```python
from build123d import *

# Parameters (mm, degrees)
F1_DEPTH = 12.7
F2_R     = 1.8288
F3_DEPTH = 5.08


# Not quite as in the source:
# - the program builds the solid bodies; features that only make, move or delete a surface that nothing else refers to are left out


with BuildPart() as f1:
    # F0 (on Top) → F1 (new body)
    with BuildSketch(Plane.XY):
        Polygon((48.4242066741, -22.2311150283), (0, 52.6062995195), (-47.3236590624, -22.2311150283), align=None)
    extrude(amount=F1_DEPTH)

    # F2 (on face) → F3 (cut)
    with BuildSketch(Plane.XY.offset(12.7)):
        with Locations((-41.0783812404, -18.9761463553)):
            Circle(F2_R)
        with Locations((-20.4600691795, -18.9761463553)):
            Circle(F2_R)
        with Locations((0, -18.9761463553)):
            Circle(F2_R)
        with Locations((19.8642425239, -18.9761463553)):
            Circle(F2_R)
        with Locations((38.6579222977, -18.9761463553)):
            Circle(F2_R)
        with Locations((-29.1365217417, 3.3634696156)):
            Circle(F2_R)
        with Locations((-11.6957994178, 3.3634696156)):
            Circle(F2_R)
        with Locations((4.2915293016, 3.3634696156)):
            Circle(F2_R)
        with Locations((22.6406212896, 3.3634696156)):
            Circle(F2_R)
        with Locations((-15.87430574, 24.0743272007)):
            Circle(F2_R)
        with Locations((0, 24.0743272007)):
            Circle(F2_R)
        with Locations((13.3752385154, 24.0743272007)):
            Circle(F2_R)
        with Locations((-5.3372029215, 40.4250063002)):
            Circle(F2_R)
        with Locations((4.2915293016, 40.4250063002)):
            Circle(F2_R)
        with Locations((0, 48.2369959354)):
            Circle(F2_R)
    extrude(amount=-F3_DEPTH, mode=Mode.SUBTRACT)


solid = f1.part
```
Can you work these out from the model? Positions are in its coordinate system, mm. A direction names the side the tool comes from. Coordinates: 2 decimals unless noted, no trailing zeros. Loops run counter-clockwise (first coordinate to the right, second up) from the corner with the lowest first, then second, coordinate; pieces in that order, holes last. Notation, with made-up numbers: M 34,77.25 L 38,77.25 A19 ccw 38,88.25 Z; hole C 85.5,-1 d10. An arc over 180 degrees is marked long. Put each result on its own line as item: value. Start each with the question number.
(1) We'd pull the mould along Y, two halves only. Please class faces 3 (the face through (20, -19, 7.62)), 4 (the face through (-0.24, 50.05, 10.2)), 5 (the face through (0, -22.231, 6)), 6 (the face through (-23.33, 15.71, 6.26)): +Y half, -Y half, draft (parallel to the pull), parting line (faces both ways), or undercut.
(2) Imagine slicing it at A-A on z = 9.5. Give the number of separate pieces and of enclosed holes in the cut face, and give its area (3 significant figures).
(3) Imagine slicing it at B-B on z = 2.5. List the corners of the cut face in (x, y) for me.
(4) Will these pins go through, and if not, where does the flat tip stop? pin 1 Ø1.8 at (x, y) = (22, 3.5) entering from +Z; pin 2 Ø4 at (x, z) = (20.5, 5) entering from +Y; pin 3 Ø2 at (y, z) = (-5, 5.5) entering from +X.
(5) Imagine slicing it at D-D on x = -36. List the corners of the cut face in (y, z) for me, and give its area (3 significant figures).
(6) Imagine slicing it at C-C on y = 37.5. List the corners of the cut face in (x, z) for me.
(7) Which directions (+Z, -Z, +X, -X, +Y, -Y) give clear straight access to the entire face, cutting with the end or side of a thin tool? Please do faces 1 (the face through (24.33, 2.66, 10.2)), 2 (the face through (0, 7, 0)).
(8) I need wall thicknesses on probe 1 along X at (y, z) = (40, 9); probe 2 along Y at (x, z) = (-27.5, 8.75); probe 3 along X at (y, z) = (2, 11.75). Which ranges of each line are inside material? Lowest first, please.
Worked answers:
1. face 3: undercut
1. face 4: undercut
1. face 5: -Y half
1. face 6: +Y half
2. separate pieces: 1
2. enclosed holes: 14
2. area: 3,430 mm2
3. outline: M -47.32,-22.23 L 48.42,-22.23 L 0,52.61 Z
4. pin 1: stops at z = 7.62
4. pin 2: stops at y = 24.02
4. pin 3: stops at x = 37.92
5. outline: M -22.23,0 L -4.32,0 L -4.32,12.7 L -22.23,12.7 Z
5. area: 227 mm2
6. outline: M -9.55,0 L 9.77,0 L 9.77,12.7 L -9.55,12.7 Z
7. face 1: +Z
7. face 2: -Z, +X, -X, +Y, -Y
8. probe 1: x = -7.97 to -7.12, -3.56 to 2.51, 6.07 to 8.16
8. probe 2: y = -22.23 to 2.55, 4.18 to 9.12
8. probe 3: x = -32 to -30.36, -27.92 to -12.91, -10.48 to 3.07, 5.51 to 21.42, 23.86 to 32.75
